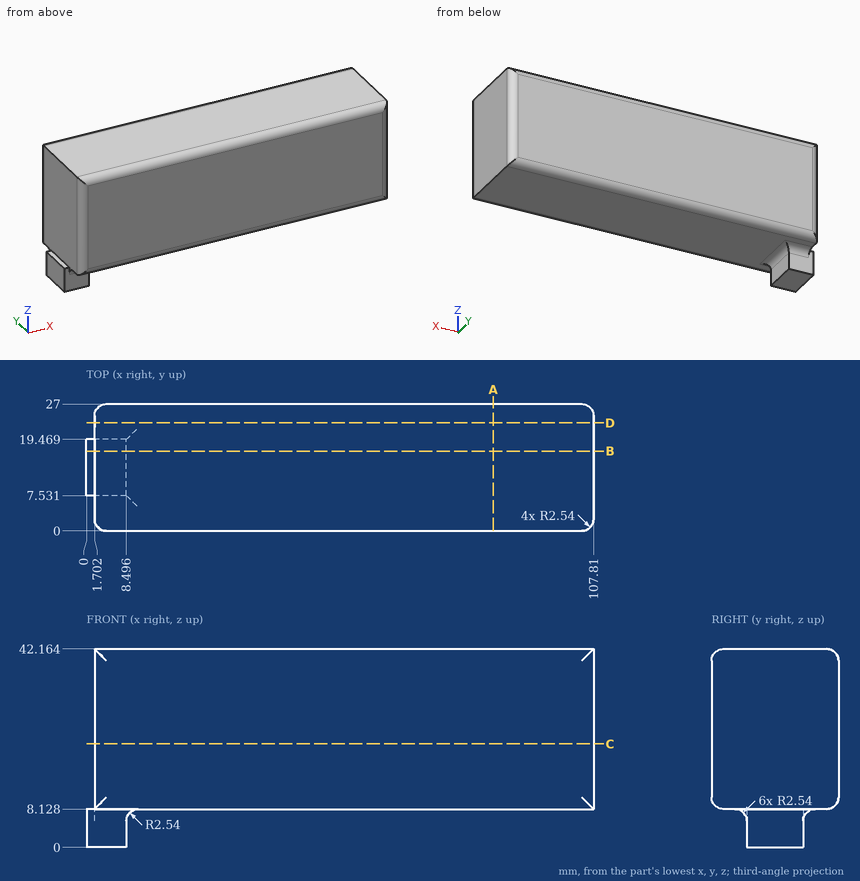
Check sheet for the drawn part. Datum: minimum x, y, z corner. Units: mm. Round coordinates to 2 decimals unless told otherwise and drop trailing zeros. Order: outer loops, then holes, each group sorted by start corner. A loop starts at its lowest first (then second) coordinate and runs counter-clockwise, first axis right, second up. Notation, with made-up numbers: M 50.25,53 L 98.25,53 A13 ccw 98.25,69 Z; hole C -17.5,-26 d10. An arc over 180 degrees is marked long. Answer in a Markdown table with one row per item.
(1) Section check B-B on y = 17. Record the boundary of the cut face in (x, z), plus the area to 3 significant figures.
Findings:
| item | result |
|---|---|
| outline | M 0,0 L 8.5,0 L 8.5,5.59 A2.54 cw 11.04,8.13 L 107.81,8.13 L 107.81,42.16 L 1.7,42.16 L 1.7,8.13 L 0,8.13 Z |
| area | 3,680 mm^2 |
(2) Gauge pin test, flat ends, axial feed: pin 1 (6 mm diameter, centred on y = 16, z = 3.5, fed in from +X); pin 2 (8 mm diameter, centred on y = 16, z = 32, fed in from -X); pin 3 (6.5 mm diameter, centred on x = 64, y = 19, fed in from -Z). Record the tip position at first contact, or that the pin passes through.
Findings:
| item | result |
|---|---|
| pin 1 | stops at x = 8.67 |
| pin 2 | stops at x = 1.7 |
| pin 3 | stops at z = 8.13 |
(3) Material ranges on line 1 along X through (y, z) = (17.5, 25); line 2 along X through (y, z) = (13.5, 4.5); line 3 along Z through (x, y) = (101.5, 24.75) (1 decimal), recorded low to high. Write a range as from..to.
Findings:
| item | result |
|---|---|
| line 1 | x = 1.7..107.81 |
| line 2 | x = 0..8.5 |
| line 3 | z = 8.1..42.1 |
(4) Section check C-C on z = 22. Record the boundary of the cut face in (x, y), plus the area to 3 significant figures.
Findings:
| item | result |
|---|---|
| outline | M 1.7,2.54 A2.54 ccw 4.24,0 L 105.27,0 A2.54 ccw 107.81,2.54 L 107.81,24.46 A2.54 ccw 105.27,27 L 4.24,27 A2.54 ccw 1.7,24.46 Z |
| area | 2,860 mm^2 |
(5) Section check D-D on y = 23. Record the boundary of the cut face in (x, z), plus the area to 3 significant figures.
Findings:
| item | result |
|---|---|
| outline | M 1.7,8.13 L 107.81,8.13 L 107.81,42.16 L 1.7,42.16 Z |
| area | 3,610 mm^2 |
(6) Section check A-A on x = 86.5. Record the boundary of the cut face in (y, z).
Findings:
| item | result |
|---|---|
| outline | M 0,10.67 A2.54 ccw 2.54,8.13 L 24.46,8.13 A2.54 ccw 27,10.67 L 27,39.62 A2.54 ccw 24.46,42.16 L 2.54,42.16 A2.54 ccw 0,39.62 Z |
